Build history of the part. All positions in model axes, mm. Round coordinates to 2 decimals unless told otherwise and drop trailing zeros. Loops run counter-clockwise (first coordinate to the right, second up) from the corner with the lowest first, then second, coordinate; pieces in that order, holes last. Notation, with made-up numbers: (47.25, 13.5) - (65.25, 13.5) arc R15 ccw to (65.25, 28.5) - close; hole circle Ø3 at (-11.5, 15.25). An arc over 180 degrees is marked (long way). Answer as CSV lines item,"result". Start each with the question number.
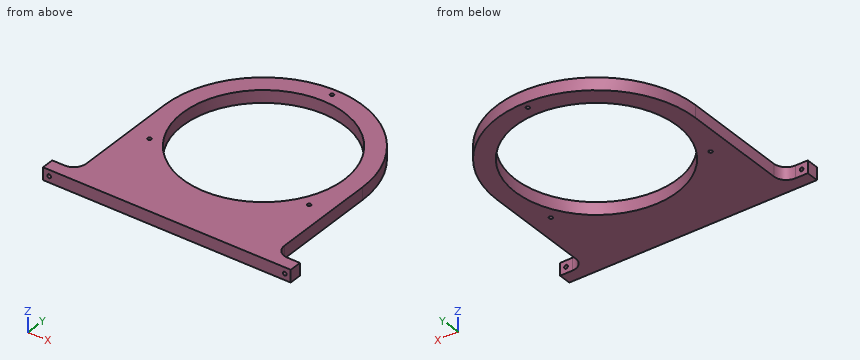
Autodesk Fusion 360 part; units mm, degrees
sketch "Sketch1" plane through (0, 0, 0) normal (0, 0, 1) x (1, 0, 0)
  circle A0 centre (0, 0) radius 65.25
  circle A1 centre (0, 0) radius 74.419 construction
  circle A2 centre (0, 74.419) radius 1.5
  circle A3 centre (-64.4487, -37.2095) radius 1.5
  circle A4 centre (64.4487, -37.2095) radius 1.5
  circle A5 centre (0, 0) radius 80
  line L0 (-80, 0) -> (80, 0) construction
  line L1 (-80, 0) -> (-80, -85)
  line L2 (80, -85) -> (80, 0)
  line L3 (-80, -95) -> (-100, -95) construction
  line L4 (-100, -95) -> (-90, -95)
  line L5 (100, -95) -> (100, -105)
  line L6 (100, -105) -> (-100, -105)
  line L7 (-100, -105) -> (-100, -95)
  arc A6 (-90, -95) -> (-80, -85) centre (-90, -85) ccw
  line L8 (90, -95) -> (100, -95)
  arc A7 (80, -85) -> (90, -95) centre (90, -85) ccw
  line L9 (-100, -100) -> (-30, -100) construction
  line L10 (-100, -100) -> (40, -100) construction
  circle A8 centre (-30, -100) radius 1.5
  circle A9 centre (40, -100) radius 1.5
  dimension "d1" = 130.5
  dimension "d4" = 148.838
  dimension "d5" = 3
  dimension "d7" = 360
  dimension "d8" = 160
  dimension "d10" = 200
  dimension "d11" = 10
  dimension "d12" = 10
  dimension "d13" = 10
  dimension "d22" = 105
  dimension "d24" = 70
  dimension "d25" = 140
  dimension "d26" = 3
  dimension "d27" = 3
extrude "Extrude1" add sketch "Sketch1" along normal blind 10 contours A5 | A5 L1 L2 L4 L5 L6 L7 A6 L8 A7 | A8 | A9
hole "Hole1" at (-95, -95, 5) direction (0, -1, 0) diameter 3 depth 10 tip angle 118
hole "Hole2" at (95.1862, -95, 5.0204) direction (0, -1, 0) diameter 3 depth 10 tip angle 118
equation "d1 = GearboxDia + Tollerance"
equation "GearboxDia = 130 mm"
equation "Tollerance = 0.5 mm"
equation "d4 = ( 74.419 * 2 ) * 1 mm"
equation "d8 = GearboxDia + 30 mm"
equation "d10 = d8 + 40 mm"
equation "d22 = AxleHieght"
equation "AxleHieght = 105 mm"
equation "d24 = ( 210 / 3 ) * 1 mm"
equation "d25 = ( 210 / 3 * 2 ) * 1 mm"
Q1. Band-saw the part on A-A, the plane y = 18.5. List the corners of the cut face in (x, z).
Q2. Wall check: probe 1 along X at (y, z) = (-101.25, 5); probe 2 along Y at (x, z) = (0, 6.5); probe 3 along Z at (x, y) = (-95, -103). Give the ranges that are in metal, low to high. Write a range as [from, to].
Q3. Band-saw the part on B-B, the plane x = 11. List the corners of the cut face in (y, z).
Q4. Pin check, flat tips, straight feed: pin 1 Ø6 at (y, z) = (-10.5, 3.5) entering from +X; pin 2 Ø1 at (y, z) = (47.5, 6.5) entering from -X; pin 3 Ø2 at (x, z) = (19.5, 2.5) entering from +Y. Stop position of each tip, or through.
Q5. Band-saw the part on C-C, the plane y = -69.5. List the corners of the cut face in (x, z), then the cut area to 3 significant figures.
Q6. Band-saw the part on D-D, the plane x = -87. List the corners of the cut face in (y, z), then the cut area to 3 significant figures.
Reported:
1,outline,"(-77.83, 0) - (-62.57, 0) - (-62.57, 10) - (-77.83, 10) - close; (62.57, 0) - (77.83, 0) - (77.83, 10) - (62.57, 10) - close"
2,probe 1,"x = [-100, -96.5], [-93.5, 93.69], [96.69, 100]"
2,probe 2,"y = [-105, -65.25], [65.25, 72.92], [75.92, 80]"
2,probe 3,"z = [0, 3.5], [6.5, 10]"
3,outline,"(-105, 0) - (-64.32, 0) - (-64.32, 10) - (-105, 10) - close; (64.32, 0) - (79.24, 0) - (79.24, 10) - (64.32, 10) - close"
4,pin 1,"stops at x = 80"
4,pin 2,"stops at x = -64.74"
4,pin 3,"stops at y = 77.83"
5,outline,"(-80, 0) - (80, 0) - (80, 10) - (-80, 10) - close"
5,area,"1,600 mm2"
6,outline,"(-105, 0) - (-94.54, 0) - (-94.54, 10) - (-105, 10) - close"
6,area,"105 mm2"
